Autodesk Inventor part; units mm, degrees
sketch "Sketch1" plane through (0, 0, 0) normal (0, 1, 0) x (-1, 0, 0)
  circle A0 centre (0, 0) radius 37.5
  circle A1 centre (0, 0) radius 25
  dimension "d0" = 75
  dimension "d1" = 50
extrude "Extrusion1" add sketch "Sketch1" along normal blind 630
sketch "Sketch2" plane through (0, 0, 0) normal (0, 1, 0) x (-1, 0, 0)
  line L0 (-37.5, -37.5) -> (37.5, -37.5)
  line L1 (37.5, -37.5) -> (37.5, 37.5)
  line L2 (37.5, 37.5) -> (-37.5, 37.5)
  line L3 (-37.5, 37.5) -> (-37.5, -37.5)
  point P0 (0, 0)
extrude "Extrusion2" add sketch "Sketch2" against normal blind 60
sketch "Sketch3" plane through (0, 0, 0) normal (0, 0, 1) x (1, 0, 0)
  circle A0 centre (0, -30) radius 15
  line L0 (-74.4823, 0) -> (79.3938, 0)
  line L1 (-37.5, 0) -> (-37.5, -60)
  line L2 (37.5, 0) -> (37.5, -60)
  arc A1 (-37.5, -30) -> (37.5, -30) centre (0, -21.5625) ccw
  line L3 (-37.5, -30) -> (-52.5, -30)
  line L4 (-52.5, -30) -> (-52.5, -80.2965)
  line L5 (-52.5, -80.2965) -> (57.4115, -80.2965)
  line L6 (57.4115, -80.2965) -> (57.4115, -30)
  line L7 (57.4115, -30) -> (37.5, -30)
  point P0 (0, 0)
  dimension "d6" = 30
  dimension "d7" = 30
extrude "Extrusion3" cut sketch "Sketch3" along normal mid plane 150 contours A0 | A1 L7 L6 L5 L4 L3
fillet "Fillet1" radius 37.5 4 edges at (37.5, -15, 37.5) (37.5, -15, -37.5) (-37.5, -15, 37.5) (-37.5, -15, -37.5)
properties part number "Cylinder_Bom"
Design review of the part built by this model. Coordinates are the model's own, in mm. Give positions to 0.01 mm unless a question says otherwise; leave off trailing zeros. Loops run counter-clockwise (first coordinate to the right, second up) from the corner with the lowest first, then second, coordinate; pieces in that order, holes last. Notation, with made-up numbers: M 65.5,3.25 L 113.5,3.25 A23 cw 113.5,39.25 Z; hole C 55.25,52 d3. An arc over 180 degrees is marked long. Write item = value, one per line.
Q1. We need section D-D (y = -7.5). Give the boundary of the cut face in (x, z).
Output values:
outline = C 0,0 d75
Q2. To check wall thickness, follow line 1 (Y direction, x = 0, z = -10); line 2 (Z direction, x = 0, y = 235.5); line 3 (Z direction, x = -2.5, y = 31). State the ranges of each line that lie inside material, in increasing order. Write a range as [from, to].
Output values:
line_1 = [-60, -45], [-15, 0]
line_2 = [-37.5, -25], [25, 37.5]
line_3 = [-37.42, -24.87], [24.87, 37.42]
Q3. We need section B-B (z = -7). Give the boundary of the cut face in (x, y) (1 decimal).
Output values:
outline = M -36.8,-32.5 A38.4 ccw 36.8,-32.5 L 36.8,630 L 24,630 L 24,0 L -24,0 L -24,630 L -36.8,630 Z; hole C 0,-30 d30
Q4. Insertion check: pin 1 (1.5 mm diameter, centred on y = 151, z = -2, fed in from -X); pin 2 (24 mm diameter, centred on x = 0, y = -30, fed in from +Z); pin 3 (4 mm diameter, centred on x = 18, y = 33, fed in from -Z); pin 4 (3 mm diameter, centred on x = -23, z = 30, fed in from -Y). Each pin has a flat end and moves straight along its axis. Give the tip position at first contact, or say it passes through.
Output values:
pin_1 = -37.48
pin_2 = through
pin_3 = -33.92
pin_4 = -53.42
Q5. We need section C-C (y = 572). Give the boundary of the cut face in (x, z), plus the area to 3 significant figures.
Output values:
outline = C 0,0 d75; hole C 0,0 d50
area = 2,450 mm^2
Q6. We need section A-A (x = -7.5). Give the boundary of the cut face in (y, z), plus the area to 3 significant figures.
Output values:
outline = M -59.26,-36.74 L -42.99,-36.74 L -42.99,36.74 L -59.26,36.74 Z; M -17.01,-36.74 L 630,-36.74 L 630,-23.85 L 0,-23.85 L 0,23.85 L 630,23.85 L 630,36.74 L -17.01,36.74 Z
area = 18,700 mm^2
Q7. Draft analysis for pull direction X (two halves, no side actions). For faces 1 (the cylindrical face through (-23.846, 310.59, -7.509)), 2 (the flat face through (-24, 630, -8)), 3 (the cylindrical face through (0.726, -59.993, -0.525)), state which applies: +X half, -X half, draft (parallel to the pull), parting line (faces both ways), or undercut.
Output values:
face_1 = undercut
face_2 = draft
face_3 = parting line
